Check sheet for the modelled part. Datum: model origin and axes. Units: mm. Face numbers are marked on the shaded views. A direction names the side the tool comes from. Give positions to 0.01 mm unless a question says otherwise; leave off trailing zeros. Loops run counter-clockwise (first coordinate to the right, second up) from the corner with the lowest first, then second, coordinate; pieces in that order, holes last. Notation, with made-up numbers: (13.5, -28.5) -> (36.5, -28.5) arc R19 ccw to (36.5, -16.5) -> close; hole circle Ø1 at (37.5, 69). An arc over 180 degrees is marked (long way). Write each question's results on one line, items separated by ' | '. Start each with the question number.
1. Gauge pin test, flat ends, axial feed: pin 1 Ø4 at (x, y) = (-3, 68.5) entering from -Z; pin 2 Ø2 at (x, y) = (-14.5, 34.5) entering from -Z; pin 3 Ø2 at (x, z) = (17.5, -5) entering from -Y; pin 4 Ø4 at (x, y) = (3, 60) entering from +Z. Record the tip position at first contact, or that the pin passes through.
2. Cross-section at C-C on x = -18. Record the boundary of the cut face in (y, z).
3. Cross-section at B-B on y = 99. Record the boundary of the cut face in (x, z).
4. Material ranges on L1, parallel to Z at x = -9, y = 63; L2, parallel to Z at x = 0, y = 87; L3, parallel to X at y = 89.5, z = 0, recorded low to high. Write a range as from..to.
5. Mould release check, pull along X, two halves, no side actions. Record for the marked faces 4, 5 and 6: +X half, -X half, draft (parallel to the pull), parting line (faces both ways), or undercut.
6. Cross-section at D-D on y = 64.5. Record the boundary of the cut face in (x, z).
7. Cross-section at A-A on z = 0. Record the boundary of the cut face in (x, y).
8. Tool access check on the marked faces 1, 2 and 3. Record the directions out of +Z, -Z, +X, -X, +Y, -Y that give a thin tool (end or side, any length) a straight path to the whole face; none if there is none.
from build123d import *

# Parameters (mm, degrees)
CUT_EXTRUDE1_DEPTH         = 114.549548656
CUT_EXTRUDE1_DEPTH_BACK    = 114.549548656
F_16_0MM_DOWEL_HOLE1_D     = 16
F_16_0MM_DOWEL_HOLE1_DEPTH = 32.693115048
F_16_0MM_DOWEL_HOLE1_TIP   = 4.806884952


with BuildPart() as part:
    # Sketch1 → Revolve1 (revolve)
    with BuildSketch(Plane(origin=(0, 0, 0), x_dir=(0, 0, -1), z_dir=(1, 0, 0))):
        Polygon((0, 0), (-22.5, 0), (-22.5, 11), (-16.5, 11), (-16.5, 84), (-12.5, 109), (0, 109), align=None)
    revolve(axis=Axis((0, 109, 0), (0, -1, 0)))

    # Sketch2 → Cut-Extrude1 (cut, two sides: drawn at the far end of the back side and taken through both)
    with BuildSketch(Plane(origin=(0, 0, 0), x_dir=(0, 0, -1), z_dir=(1, 0, 0)).offset(-CUT_EXTRUDE1_DEPTH_BACK)):
        with BuildLine():
            Line((-9, 37), (-9, 67))
            ThreePointArc((-9, 67), (0, 76), (9, 67))
            Line((9, 67), (9, 37))
            ThreePointArc((9, 37), (0, 28), (-9, 37))
        make_face()
    extrude(amount=CUT_EXTRUDE1_DEPTH + CUT_EXTRUDE1_DEPTH_BACK, mode=Mode.SUBTRACT)

    # Ø16.0mm Dowel Hole1
    with Locations(Plane.ZX.offset(109)):
        with Locations((0, 0)):
            Hole(F_16_0MM_DOWEL_HOLE1_D / 2, depth=F_16_0MM_DOWEL_HOLE1_DEPTH)
            with Locations((0, 0, -(F_16_0MM_DOWEL_HOLE1_DEPTH + F_16_0MM_DOWEL_HOLE1_TIP / 2))):  # 118° drill point
                Cone(0, F_16_0MM_DOWEL_HOLE1_D / 2, F_16_0MM_DOWEL_HOLE1_TIP, mode=Mode.SUBTRACT)


solid = part.part
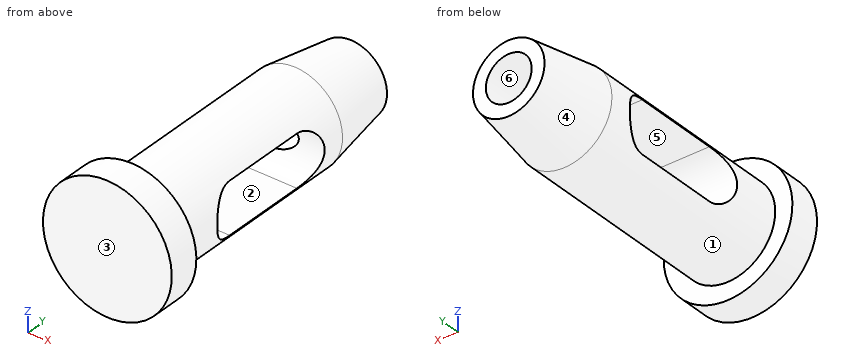
Geometry says:
1) pin 1: z = -16.47 | pin 2: z = -9.49 | pin 3: y = 0 | pin 4: z = 16.47
2) outline: (0, -13.5) -> (11, -13.5) -> (11, 13.5) -> (0, 13.5) -> close
3) outline: circle Ø28.2 at (0, 0); hole circle Ø16 at (0, 0)
4) L1: -13.83..-9, 9..13.83 | L2: -16.02..-8, 8..16.02 | L3: -15.62..-8, 8..15.62
5) face 4: parting line | face 5: draft | face 6: undercut
6) outline: (-13.83, -9) arc R16.5 ccw to (13.83, -9) -> close; (-13.83, 9) -> (13.83, 9) arc R16.5 ccw to start
7) outline: (-22.5, 0) -> (22.5, 0) -> (22.5, 11) -> (16.5, 11) -> (16.5, 28) -> (-16.5, 28) -> (-16.5, 11) -> (-22.5, 11) -> close; (-16.5, 76) -> (-7.49, 76) -> (-8, 76.31) -> (-8, 109) -> (-12.5, 109) -> (-16.5, 84) -> close; (7.49, 76) -> (16.5, 76) -> (16.5, 84) -> (12.5, 109) -> (8, 109) -> (8, 76.31) -> close
8) face 1: +Y | face 2: +X, -X | face 3: +Z, -Z, +X, -X, -Y
